```python
from build123d import *

# Parameters (mm, degrees)
F0_R     = 37.5
F1_DEPTH = 2.5


with BuildPart() as f1:
    # F0 (on Front) → F1 (new body, symmetric)
    with BuildSketch(Plane.XZ):
        with BuildLine():
            ThreePointArc((23.495791584, -34.5144310796), (-2.7972530191, -27.5212402414), (-27.9439404953, -37.9074340379))
            ThreePointArc((-27.9439404953, -37.9074340379), (-17.5873893593, -108.6193138327), (42.5, -69.9290859253))
            ThreePointArc((42.5, -69.9290859253), (37.4487726255, -49.8333294369), (23.495791584, -34.5144310796))
        make_face()
        with Locations((0, -69.9290859253)):
            Circle(F0_R, mode=Mode.SUBTRACT)
        with BuildLine():
            add(Edge.make_bspline(
                [(5.1920566863, 18.5723408589), (5.4030836199, 18.1737175795), (6.009346047, 17.0894557175), (8.4647401185, 15.2993210086), (10.0607038312, 14.1674244584)],
                knots=[0, 0, 0, 0, 0.353980682, 1, 1, 1, 1], degree=3))
            ThreePointArc((5.1920566863, 18.5723408589), (0, 22.4882426928), (-5.1920566863, 18.5723408589))
            add(Edge.make_bspline(
                [(-5.1920566863, 18.5723408589), (-5.4030836199, 18.1737175795), (-6.009346047, 17.0894557175), (-8.4647401185, 15.2993210086), (-10.0607038312, 14.1674244584)],
                knots=[0, 0, 0, 0, 0.353980682, 1, 1, 1, 1], degree=3))
            ThreePointArc((-10.0607038312, 14.1674244584), (-16.0703171245, 6.6420670409), (-17.1570047894, -2.9269227761))
            ThreePointArc((-17.1570047894, -2.9269227761), (-16.488459767, -3.9392853203), (-15.2897240847, -4.1260020361))
            ThreePointArc((-15.2897240847, -4.1260020361), (-14.4157806287, -3.4876204113), (-14.1989005153, -2.4273038173))
            ThreePointArc((-14.1989005153, -2.4273038173), (-12.2569494075, 7.5291203707), (-4.2325370023, 13.7347921529))
            ThreePointArc((-4.2325370023, 13.7347921529), (-3.0879498251, 15.2971102039), (-2.3815860794, 17.1004315168))
            ThreePointArc((-2.3815860794, 17.1004315168), (-2.3733660378, 17.1550903584), (-2.3638894327, 17.2095454042))
            ThreePointArc((-2.3638894327, 17.2095454042), (-0.0049388321, 19.1708665497), (2.3550204808, 17.2107592534))
            ThreePointArc((2.3550204808, 17.2107592534), (3.060795291, 15.3469315093), (4.2325370023, 13.7347921529))
            ThreePointArc((4.2325370023, 13.7347921529), (13.9491841539, 3.5458163369), (10.330929233, -10.0606781189))
            add(Edge.make_bspline(
                [(10.330929233, -10.0606781189), (7.0163060906, -15.4310663182), (0.8325115992, -23.801862272), (-9.7668403245, -26.9773220336), (-21.5660588981, -32.3417266701), (-27.9439404953, -37.9074340379)],
                knots=[0, 0, 0, 0, 0.3399679741, 0.609879003, 1, 1, 1, 1], degree=3))
            ThreePointArc((-27.9439404953, -37.9074340379), (-2.7972530191, -27.5212402414), (23.495791584, -34.5144310796))
            add(Edge.make_bspline(
                [(15.4707114186, -7.9926174921), (14.2001866213, -13.2718644657), (11.6427356628, -23.7542991739), (19.5641259536, -30.9373140161), (23.495791584, -34.5144310796)],
                knots=[0, 0, 0, 0, 0.5020174455, 1, 1, 1, 1], degree=3))
            ThreePointArc((15.4707114186, -7.9926174921), (16.9035545368, 4.0975903429), (10.0607038312, 14.1674244584))
        make_face()
        with BuildLine():
            ThreePointArc((-2.3638894327, 17.2095454042), (-2.3733660378, 17.1550903584), (-2.3815860794, 17.1004315168))
            ThreePointArc((-2.3815860794, 17.1004315168), (-2.3680946087, 17.1555451395), (-2.3550204808, 17.2107592534))
            ThreePointArc((-2.3550204808, 17.2107592534), (-2.3594550348, 17.2101528992), (-2.3638894327, 17.2095454042))
        make_face()
    extrude(amount=F1_DEPTH, both=True)


solid = f1.part
```
Check sheet for the modelled part. Datum: model origin and axes. Units: mm. A direction names the side the tool comes from. Round coordinates to 2 decimals unless told otherwise and drop trailing zeros. Loops run counter-clockwise (first coordinate to the right, second up) from the corner with the lowest first, then second, coordinate; pieces in that order, holes last. Notation, with made-up numbers: (-27, 38.25) - (-9, 38.25) arc R20 cw to (-9, 45.25) - close; hole circle Ø9 at (81.5, -25). An arc over 180 degrees is marked (long way). Answer as a JSON object with one key per item and string values. Group by question number.
Q1. Sectioned sample at B-B, the plane x = 32. Enter the section's corners in (y, z), plus the area to 3 significant figures.
Q2. Sectioned sample at A-A, the plane z = -64. Enter the section's corners in (x, y), plus the area to 3 significant figures.
Q3. Gauge pin test, flat ends, axial feed: P1, Ø2, axis at y = 0.5, z = -64, coming from the -X side; P2, Ø2, axis at x = -23, y = 0, coming from the +Z side; P3, Ø1.5, axis at y = -1, z = -13, coming from the -X side; P4, Ø10, axis at x = -12, z = -38.5, coming from the +Y side. Record the tip position at first contact, or that the pin passes through.
Q4. Sectioned sample at C-C, the plane x = -11.5. Count the separate pieces of the cut face and the enclosed holes in it, plus the area to 3 significant figures.
Q5. Scan lines: line 1 along Z through (x, y) = (-6.5, 1.4); line 2 along Z through (x, y) = (6, -0.3); line 3 along X through (y, z) = (-0.7, 0). Record each from-to range of solid material in increasing order. Write a range as [from, to].
Q6. Set-up check for faces 5 (the face through (0, 2.5, -30)), 6 (the face through (-0.05, -0.04, 19.17)): record each of +Z, -Z, +X, -X, +Y, -Y from which the full face is reachable in a straight line by a thin tool's end or side.
Q7. Mould release check, pull along X, two halves, no side actions. Record for faces 1 (the face through (16.944, -0.035, 3.928)), 2 (the face through (1.32, -0.04, -112.41)), 3 (the face through (-16.017, -0.035, 6.768)), 4 (the face through (3.05, -0.04, 15.37)): released by +X, released by -X, zero draft, split by the parting line, or undercut.
Solution:
{
 "1": {"outline": "(-2.5, -97.9) - (2.5, -97.9) - (2.5, -89.48) - (-2.5, -89.48) - close; (-2.5, -50.38) - (2.5, -50.38) - (2.5, -41.96) - (-2.5, -41.96) - close", "area": "84.2 mm²"},
 "2": {"outline": "(-42.08, -2.5) - (-37.03, -2.5) - (-37.03, 2.5) - (-42.08, 2.5) - close; (37.03, -2.5) - (42.08, -2.5) - (42.08, 2.5) - (37.03, 2.5) - close", "area": "50.6 mm²"},
 "3": {"P1": "stops at x = -42.21", "P2": "stops at z = -33.44", "P3": "stops at x = 7.95", "P4": "stops at y = 2.5"},
 "4": {"separate pieces": "3", "enclosed holes": "0", "area": "79.2 mm²"},
 "5": {"line 1": "z = [-111.93, -106.86], [-33, -26.09], [12.82, 16.89]", "line 2": "z = [-112, -106.95], [-32.91, -16.48], [13.06, 17.39]", "line 3": "x = [-17.4, -14.4], [14.4, 17.4]"},
 "6": {"face 5": "+Z, -Z, +X, -X, +Y", "face 6": "+Y, -Y"},
 "7": {"face 1": "released by +X", "face 2": "split by the parting line", "face 3": "released by -X", "face 4": "undercut"}
}
